```python
from build123d import *

# Parameters (mm, degrees)
ESQUISSE1_W                = 31.939489742
ESQUISSE1_H                = 21.744204364
ESQUISSE1_R                = 1
BOSS_EXTRU_1_DEPTH         = 5
ESQUISSE2_R                = 2.5
ESQUISSE2_R_2              = 1
BOSS_EXTRU_2_DEPTH         = 2.5
ESQUISSE4_R                = 1.5
BOSS_EXTRU_3_DEPTH         = 5
R_P_TITION_LIN_AIRE1_COUNT = 2
R_P_TITION_LIN_AIRE1_PITCH = 27


with BuildPart() as part:
    # Esquisse1 → Boss.-Extru.1 (new body)
    with BuildSketch(Plane.XY):
        with Locations((0, -1.253300442)):
            Rectangle(ESQUISSE1_W, ESQUISSE1_H)
        with Locations((10.5, 6.25)):
            Circle(ESQUISSE1_R, mode=Mode.SUBTRACT)
        with Locations((10.5, -6.25)):
            Circle(ESQUISSE1_R, mode=Mode.SUBTRACT)
        with Locations((-10.5, -6.25)):
            Circle(ESQUISSE1_R, mode=Mode.SUBTRACT)
        with Locations((-10.5, 6.25)):
            Circle(ESQUISSE1_R, mode=Mode.SUBTRACT)
    extrude(amount=BOSS_EXTRU_1_DEPTH)

    # Esquisse2 → Boss.-Extru.2 (add)
    # profile 1 of 4: a face of its own
    with BuildSketch(Plane.XY.offset(5)):
        with Locations(Location((-10.5, 6.25, 0), (0, 0, 180))):
            Circle(ESQUISSE2_R)
        with Locations((-10.5, 6.25)):
            Circle(ESQUISSE2_R_2, mode=Mode.SUBTRACT)
    # profile 2 of 4: a face of its own
    with BuildSketch(Plane.XY.offset(5)):
        with Locations(Location((10.5, 6.25, 0), (0, 0, 180))):
            Circle(ESQUISSE2_R)
        with Locations((10.5, 6.25)):
            Circle(ESQUISSE2_R_2, mode=Mode.SUBTRACT)
    # profile 3 of 4: a face of its own
    with BuildSketch(Plane.XY.offset(5)):
        with Locations(Location((10.5, -6.25, 0), (0, 0, 180))):
            Circle(ESQUISSE2_R)
        with Locations((10.5, -6.25)):
            Circle(ESQUISSE2_R_2, mode=Mode.SUBTRACT)
    # profile 4 of 4: a face of its own
    with BuildSketch(Plane.XY.offset(5)):
        with Locations(Location((-10.5, -6.25, 0), (0, 0, 180))):
            Circle(ESQUISSE2_R)
        with Locations((-10.5, -6.25)):
            Circle(ESQUISSE2_R_2, mode=Mode.SUBTRACT)
    extrude(amount=BOSS_EXTRU_2_DEPTH)

    # Esquisse4 → Boss.-Extru.3 (add)
    with BuildSketch(Plane.ZY.offset(15.969744871)):
        with BuildLine():
            Line((0, -4.091257207), (-5.5, -4.091257207))
            ThreePointArc((-5.5, -4.091257207), (-6.560660172, -3.651917379), (-7, -2.591257207))
            Line((-7, -2.591257207), (-7, 2.408742793))
            ThreePointArc((-7, 2.408742793), (-6.560660172, 3.469402965), (-5.5, 3.908742793))
            Line((-5.5, 3.908742793), (0, 3.908742793))
            Line((0, 3.908742793), (0, -4.091257207))
        make_face()
        with Locations((-3.5, -0.091257207)):
            Circle(ESQUISSE4_R, mode=Mode.SUBTRACT)
    boss_extru_3 = extrude(amount=-BOSS_EXTRU_3_DEPTH)

    # Répétition linéaire1: Boss.-Extru.3 ×2
    with Locations(*[(i * R_P_TITION_LIN_AIRE1_PITCH, 0, 0) for i in range(1, R_P_TITION_LIN_AIRE1_COUNT)]):
        add(boss_extru_3)


solid = part.part
```
Model file for the job. Use its own axes, mm. A direction names the side the tool comes from. Coordinates: 2 decimals unless noted, no trailing zeros. Loops run counter-clockwise (first coordinate to the right, second up) from the corner with the lowest first, then second, coordinate; pieces in that order, holes last. Notation, with made-up numbers: M 80,42 L 88,42 A14 ccw 88,51 Z; hole C 4.25,10.5 d6. An arc over 180 degrees is marked long. Use CSV: the item, a comma, the result in double quotes. Start each with the question number.
1. Flat gauge pins, fed straight in: pin 1 (1 mm diameter, centred on x = -8.5, y = -1, fed in from +Z); pin 2 (2.5 mm diameter, centred on x = -10.5, y = 6.25, fed in from -Z); pin 3 (4 mm diameter, centred on x = -14, z = -2.5, fed in from -Y). Where does each tip first touch, or does it go through?
2. Band-saw the part on D-D, the plane z = 2.75. List the corners of the cut face in (x, y), then the cut area to 3 significant figures.
3. Band-saw the part on C-C, the plane y = -6.25. List the corners of the cut face in (x, z), then the cut area to 3 significant figures.
4. Tool access for faces 4 (the flat face through (15.97, -1, 2)), 5 (the flat face through (-14, 3.909, -3)), 6 (the flat face through (13, -4.091, -3)), 7 (the cylindrical face through (12.998, -6.36, 6.232)): list every direction of +Z, -Z, +X, -X, +Y, -Y with a clear straight run to the whole face (end or side of a thin tool).
5. Band-saw the part on B-B, the plane z = 6.5. List the corners of the cut face in (x, y).
6. Probe probe 1 along Y at (x, z) = (-10.5, 4.25); probe 2 along X at (y, z) = (-3.5, -4.75); probe 3 along Z at (x, y) = (-1, 5). List the from-to ranges inside material, lowest first. Write a range as [from, to].
7. Two-plate mould, pull along X, no slides. Class faces 1 (the flat face through (-15.97, -1, 0)), 2 (the flat face through (13, 3.909, -3)), 3 (the flat face through (0, -1, 0)): pulls with the +X half, pulls with the -X half, needs draft (parallel to the pull), parting line crosses it, or undercut.
8. Band-saw the part on A-A, the plane x = 10.5. List the corners of the cut face in (y, z).
Entries:
1,pin 1,"stops at z = 5"
1,pin 2,"stops at z = 0"
1,pin 3,"stops at y = -4.09"
2,outline,"M -15.97,-12.13 L 15.97,-12.13 L 15.97,9.62 L -15.97,9.62 Z; hole C -10.5,-6.25 d2; hole C -10.5,6.25 d2; hole C 10.5,-6.25 d2; hole C 10.5,6.25 d2"
2,area,"682 mm2"
3,outline,"M -15.97,0 L -11.5,0 L -11.5,7.5 L -13,7.5 L -13,5 L -15.97,5 Z; M -9.5,0 L 9.5,0 L 9.5,7.5 L 8,7.5 L 8,5 L -8,5 L -8,7.5 L -9.5,7.5 Z; M 11.5,0 L 15.97,0 L 15.97,5 L 13,5 L 13,7.5 L 11.5,7.5 Z"
3,area,"155 mm2"
4,face 4,"+Z, +X, +Y, -Y"
4,face 5,"-Z, +X, -X, +Y"
4,face 6,"-Z, +X, -X, -Y"
4,face 7,"+Z"
5,outline,"C -10.5,-6.25 d5; C -10.5,6.25 d5; C 10.5,-6.25 d5; C 10.5,6.25 d5; hole C -10.5,-6.25 d2; hole C -10.5,6.25 d2; hole C 10.5,-6.25 d2; hole C 10.5,6.25 d2"
6,probe 1,"y = [-12.13, -7.25], [-5.25, 5.25], [7.25, 9.62]"
6,probe 2,"x = [-15.97, -10.97], [11.03, 16.03]"
6,probe 3,"z = [0, 5]"
7,face 1,"pulls with the -X half"
7,face 2,"needs draft"
7,face 3,"undercut"
8,outline,"M -12.13,0 L -7.25,0 L -7.25,7.5 L -8.75,7.5 L -8.75,5 L -12.13,5 Z; M -5.25,0 L 5.25,0 L 5.25,7.5 L 3.75,7.5 L 3.75,5 L -3.75,5 L -3.75,7.5 L -5.25,7.5 Z; M 7.25,0 L 9.62,0 L 9.62,5 L 8.75,5 L 8.75,7.5 L 7.25,7.5 Z"
